from build123d import *

# Parameters (mm, degrees)
SKETCH1_W                                  = 95.25
SKETCH1_H                                  = 44.45
BOSS_EXTRUDE1_DEPTH                        = 3.175
SKETCH2_W                                  = 95.25
SKETCH2_H                                  = 44.45
SKETCH2_W_2                                = 88.9
SKETCH2_H_2                                = 38.1
BOSS_EXTRUDE2_DEPTH                        = 28.9
SKETCH3_R                                  = 1.7
CUT_EXTRUDE1_DEPTH                         = 62.570259663
CUT_EXTRUDE2_DEPTH                         = 1.7145
FILLET1_R                                  = 1.5875
BOSS_EXTRUDE3_START                        = 1.5875
BOSS_EXTRUDE3_DEPTH                        = 1.5875
SKETCH6_R                                  = 1.715
BOSS_EXTRUDE4_DEPTH                        = 19.05
SKETCH7_R                                  = 1.715
CUT_EXTRUDE3_DEPTH                         = 58.061737399
CUT_EXTRUDE4_DEPTH                         = 1.7145
MIRROR3_AT_THE_SECOND_PLANE_COPY_1_SKETC_R = 1.715
MIRROR3_AT_THE_SECOND_PLANE_COPY_1_DEPTH   = 19.05
MIRROR3_AT_THE_SECOND_PLANE_COPY_2_SKETC_R = 1.715
MIRROR3_AT_THE_SECOND_PLANE_COPY_2_DEPTH   = 58.061737399
MIRROR3_AT_THE_SECOND_PLANE_COPY_3_DEPTH   = 1.7145
SKETCH9_R                                  = 1.59
CUT_EXTRUDE5_DEPTH                         = 101.523231923


with BuildPart() as part:
    # Sketch1 → Boss-Extrude1 (new body)
    with BuildSketch(Plane.XY):
        Rectangle(SKETCH1_W, SKETCH1_H)
    extrude(amount=BOSS_EXTRUDE1_DEPTH)

    # Sketch2 → Boss-Extrude2 (add)
    with BuildSketch(Plane.XY.offset(3.175)):
        Rectangle(SKETCH2_W, SKETCH2_H)
        Rectangle(SKETCH2_W_2, SKETCH2_H_2, mode=Mode.SUBTRACT)
    extrude(amount=BOSS_EXTRUDE2_DEPTH)

    # Sketch3 → Cut-Extrude1 (cut, through all)
    with BuildSketch(Plane(origin=(0, 0, 0), x_dir=(-1, 0, 0), z_dir=(0, 0, -1))):
        with Locations((27.051, 0)):
            Circle(SKETCH3_R)
    cut_extrude1 = extrude(amount=-CUT_EXTRUDE1_DEPTH, mode=Mode.SUBTRACT)

    # Mirror1: Cut-Extrude1 across plane
    add(cut_extrude1.mirror(Plane(origin=(0, 0, 0), x_dir=(0, 0, 1), z_dir=(1, 0, 0))), mode=Mode.SUBTRACT)

    # Sketch4 → Cut-Extrude2 (cut)
    with BuildSketch(Plane(origin=(0, 0, 0), x_dir=(-1, 0, 0), z_dir=(0, 0, -1))):
        Polygon((30.497781106, 0), (28.774390553, 2.984999999), (25.327609447, 2.984999999), (23.604218894, 0), (25.327609447, -2.984999999), (28.774390553, -2.984999999), align=None)
    cut_extrude2 = extrude(amount=-CUT_EXTRUDE2_DEPTH, mode=Mode.SUBTRACT)

    # Mirror2: Cut-Extrude2 across plane
    add(cut_extrude2.mirror(Plane(origin=(0, 0, 0), x_dir=(0, 0, 1), z_dir=(1, 0, 0))), mode=Mode.SUBTRACT)

    # Fillet1
    fillet1_edges = [part.edges().sort_by_distance(p)[0] for p in [
        (44.45, 19.05, 17.625),
        (-44.45, 19.05, 17.625),
        (-44.45, -19.05, 17.625),
        (44.45, -19.05, 17.625),
        (47.625, -22.225, 16.0375),
        (-47.625, -22.225, 16.0375),
        (-47.625, 22.225, 16.0375),
        (47.625, 22.225, 16.0375),
    ]]
    fillet(fillet1_edges, radius=FILLET1_R)

    # Sketch5 → Boss-Extrude3 (add)
    with BuildSketch(Plane.XY.offset(32.075).offset(BOSS_EXTRUDE3_START)):
        with BuildLine():
            Line((-44.323, -20.5105), (44.323, -20.5105))
            ThreePointArc((44.323, -20.5105), (45.445532015, -20.045532015), (45.9105, -18.923))
            Line((45.9105, -18.923), (45.9105, 18.923))
            ThreePointArc((45.9105, 18.923), (45.445532015, 20.045532015), (44.323, 20.5105))
            Line((44.323, 20.5105), (-44.323, 20.5105))
            ThreePointArc((-44.323, 20.5105), (-45.445532015, 20.045532015), (-45.9105, 18.923))
            Line((-45.9105, 18.923), (-45.9105, -18.923))
            ThreePointArc((-45.9105, -18.923), (-45.445532015, -20.045532015), (-44.323, -20.5105))
        make_face()
        with BuildLine():
            Line((44.45, -17.4625), (44.45, 17.4625))
            ThreePointArc((44.45, 17.4625), (43.985032015, 18.585032015), (42.8625, 19.05))
            Line((42.8625, 19.05), (-42.8625, 19.05))
            ThreePointArc((-42.8625, 19.05), (-43.985032015, 18.585032015), (-44.45, 17.4625))
            Line((-44.45, 17.4625), (-44.45, -17.4625))
            ThreePointArc((-44.45, -17.4625), (-43.985032015, -18.585032015), (-42.8625, -19.05))
            Line((-42.8625, -19.05), (42.8625, -19.05))
            ThreePointArc((42.8625, -19.05), (43.985032015, -18.585032015), (44.45, -17.4625))
        make_face(mode=Mode.SUBTRACT)
    extrude(amount=-BOSS_EXTRUDE3_DEPTH)

    # Sketch6 → Boss-Extrude4 (add)
    with BuildSketch(Plane.XY.offset(3.175)):
        with BuildLine():
            Line((-44.45, 19.05), (-38.1, 19.05))
            Line((-38.1, 19.05), (-38.1, 14.2875))
            ThreePointArc((-38.1, 14.2875), (-38.564967985, 13.164967985), (-39.6875, 12.7))
            Line((-39.6875, 12.7), (-44.45, 12.7))
            Line((-44.45, 12.7), (-44.45, 19.05))
        make_face()
        with Locations(Location((-41.275, 15.875, 0), (0, 0, 180))):
            Circle(SKETCH6_R, mode=Mode.SUBTRACT)
    boss_extrude4 = extrude(amount=BOSS_EXTRUDE4_DEPTH)

    # Sketch7 → Cut-Extrude3 (cut, through all)
    with BuildSketch(Plane.XY.offset(22.225)):
        with Locations(Location((-41.275, 15.875, 0), (0, 0, 180))):
            Circle(SKETCH7_R)
    cut_extrude3 = extrude(amount=-CUT_EXTRUDE3_DEPTH, mode=Mode.SUBTRACT)

    # Sketch8 → Cut-Extrude4 (cut)
    with BuildSketch(Plane(origin=(0, 0, 0), x_dir=(-1, 0, 0), z_dir=(0, 0, -1))):
        Polygon((37.828218893, 15.875), (39.551609446, 12.89), (42.998390554, 12.89), (44.721781107, 15.875), (42.998390554, 18.86), (39.551609446, 18.86), align=None)
    cut_extrude4 = extrude(amount=-CUT_EXTRUDE4_DEPTH, mode=Mode.SUBTRACT)

    # Mirror3: Boss-Extrude4, Cut-Extrude3, Cut-Extrude4 across plane
    add(boss_extrude4.mirror(Plane(origin=(0, 0, 0), x_dir=(0, 0, 1), z_dir=(1, 0, 0))))
    add(cut_extrude3.mirror(Plane(origin=(0, 0, 0), x_dir=(0, 0, 1), z_dir=(1, 0, 0))), mode=Mode.SUBTRACT)
    add(cut_extrude4.mirror(Plane(origin=(0, 0, 0), x_dir=(0, 0, 1), z_dir=(1, 0, 0))), mode=Mode.SUBTRACT)

    # Mirror3 at the second plane: Boss-Extrude4, Cut-Extrude3, Cut-Extrude4 across plane
    add(boss_extrude4.mirror(Plane.ZX))
    add(cut_extrude3.mirror(Plane.ZX), mode=Mode.SUBTRACT)
    add(cut_extrude4.mirror(Plane.ZX), mode=Mode.SUBTRACT)

    # Mirror3 at the second plane copy 1 sketc → Mirror3 at the second plane copy 1 (add)
    with BuildSketch(Plane(origin=(0, 0, 3.175), x_dir=(-1, 0, 0), z_dir=(0, 0, 1))):
        with BuildLine():
            Line((-44.45, 19.05), (-38.1, 19.05))
            Line((-38.1, 19.05), (-38.1, 14.2875))
            ThreePointArc((-38.1, 14.2875), (-38.564967985, 13.164967985), (-39.6875, 12.7))
            Line((-39.6875, 12.7), (-44.45, 12.7))
            Line((-44.45, 12.7), (-44.45, 19.05))
        make_face()
        with Locations(Location((-41.275, 15.875, 0), (0, 0, 180))):
            Circle(MIRROR3_AT_THE_SECOND_PLANE_COPY_1_SKETC_R, mode=Mode.SUBTRACT)
    extrude(amount=MIRROR3_AT_THE_SECOND_PLANE_COPY_1_DEPTH)

    # Mirror3 at the second plane copy 2 sketc → Mirror3 at the second plane copy 2 (cut, through all)
    with BuildSketch(Plane(origin=(0, 0, 22.225), x_dir=(-1, 0, 0), z_dir=(0, 0, 1))):
        with Locations(Location((-41.275, 15.875, 0), (0, 0, 180))):
            Circle(MIRROR3_AT_THE_SECOND_PLANE_COPY_2_SKETC_R)
    extrude(amount=-MIRROR3_AT_THE_SECOND_PLANE_COPY_2_DEPTH, mode=Mode.SUBTRACT)

    # Mirror3 at the second plane copy 3 sketc → Mirror3 at the second plane copy 3 (cut)
    with BuildSketch(Plane(origin=(0, 0, 0), x_dir=(1, 0, 0), z_dir=(0, 0, -1))):
        Polygon((37.828218893, 15.875), (39.551609446, 12.89), (42.998390554, 12.89), (44.721781107, 15.875), (42.998390554, 18.86), (39.551609446, 18.86), align=None)
    extrude(amount=-MIRROR3_AT_THE_SECOND_PLANE_COPY_3_DEPTH, mode=Mode.SUBTRACT)

    # Sketch9 → Cut-Extrude5 (cut, through all)
    with BuildSketch(Plane.ZY.offset(-44.45)):
        with Locations((15.875, 0)):
            Circle(SKETCH9_R)
    extrude(amount=-CUT_EXTRUDE5_DEPTH, mode=Mode.SUBTRACT)


solid = part.part
Read the model definition and answer for the solid it produces. Units are mm, in the model's axes. A direction names the side the tool comes from. Round coordinates to 2 decimals unless told otherwise and drop trailing zeros.
Q1. Each of these flat-tipped pins is pushed along its axis until it touches: pin 1 (12 mm diameter, centred on x = -9, y = -6.5, fed in from -Z); pin 2 (3 mm diameter, centred on x = 41.275, y = -15.875, fed in from -Z); pin 3 (1.8 mm diameter, centred on x = 42, y = 17, fed in from -Z); pin 4 (2 mm diameter, centred on x = 13, y = 3.5, fed in from +Z) (3 decimals). Where does it stop, or does it pass through?
Q2. Consider probe 1 along Y at (x, z) = (-38, 11) (3 decimals); probe 2 along X at (y, z) = (-10, 32) (3 decimals); probe 3 along Y at (x, z) = (-41.5, 13) (3 decimals). Determine where each line is inside the solid, lowest interval first.
Q3. Which of the six approach directions +Z, -Z, +X, -X, +Y, -Y give full straight-line access (tool end or side, diameter ignored) to faces 5 (the face through (40.9, 17.55, 11.83)), 6 (the face through (38.1, -17, 13)), 7 (the face through (46.015, -0.967, 14.613)), 8 (the face through (-43.848, 14.362, 0.845))?
Q4. Section A-A on z = 13 is taken. Give the number of separate pieces and of enclosed holes in the cut face, and give its area (3 significant figures).
Q5. Determine the mould class of faces 1 (the face through (47.625, 0, 19)), 2 (the face through (-1, 22.225, 16)), 3 (the face through (-47.625, 0, 16)), 4 (the face through (-43.9, -17.3, 0.8)) for opening direction X: released by +X, released by -X, zero draft, split by the parting line, or undercut.
Output:
1. pin 1: stops at z = 0
1. pin 2: passes through
1. pin 3: stops at z = 1.71
1. pin 4: stops at z = 3.175
2. probe 1: y = -22.225 to -19.05, 19.05 to 22.225
2. probe 2: x = -47.625 to -44.45, 44.45 to 47.625
2. probe 3: y = -22.225 to -17.575, -14.175 to -12.7, 12.7 to 14.175, 17.575 to 22.225
3. face 5: +Z, -Z
3. face 6: +Z
3. face 7: +X
3. face 8: -Z
4. separate pieces: 1
4. enclosed holes: 5
4. area: 967 mm2
5. face 1: released by +X
5. face 2: zero draft
5. face 3: released by -X
5. face 4: undercut
